Answer from the drawing. Dimensions are ordinates in mm from the lowest x, y and z of the part. Give positions to 0.01 mm unless a question says otherwise; leave off trailing zeros. Write each loop counter-clockwise with the first axis right and the second up, starting at its lowest first coordinate (ties: lowest second). Pieces come first, ordered by that corner, then holes. Notation, with made-up numbers: (-14, -8) -> (42, -8) arc R23 ccw to (42, 14) -> close; hole circle Ø3 at (-38.5, 51.5). An arc over 180 degrees is marked (long way). Write item = value, one per line.
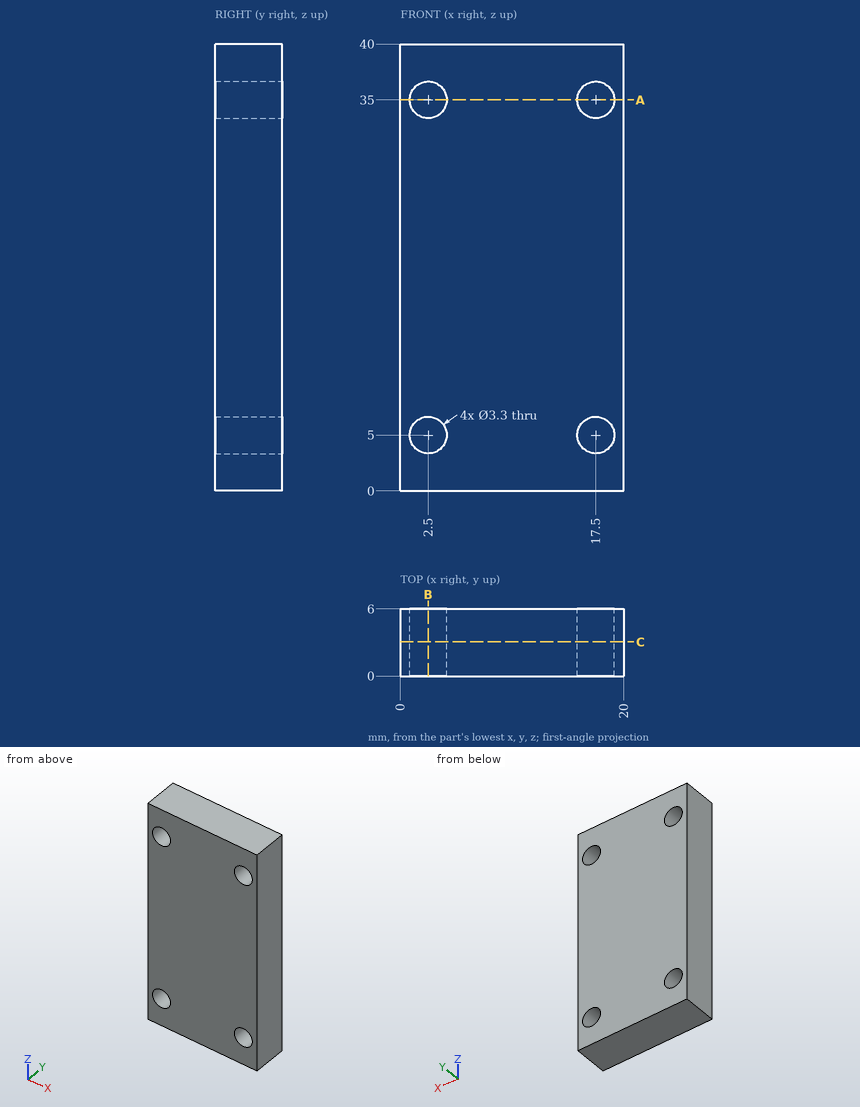
(1) Given P1, Ø8, axis at x = 4, z = 33, coming from the -Y side, flat-ended and moving along its own axis, determine where the tip first touches the part or whether it passes through.
Checks:
P1 = 0
(2) Consider L1, parallel to Z at x = 2.5, y = 3.3; L2, parallel to Z at x = 3.75, y = 4.45; L3, parallel to X at y = 3.95, z = 5.5. Determine where each line is inside the solid, lowest interval first.
Checks:
L1 = 0 to 3.35, 6.65 to 33.35, 36.65 to 40
L2 = 0 to 3.92, 6.08 to 33.92, 36.08 to 40
L3 = 0 to 0.93, 4.07 to 15.93, 19.07 to 20
(3) The part is cut by section A-A on z = 35. Determine the outline of the cut face in (x, y), plus the area to 3 significant figures.
Checks:
outline = (0, 0) -> (0.85, 0) -> (0.85, 6) -> (0, 6) -> close; (4.15, 0) -> (15.85, 0) -> (15.85, 6) -> (4.15, 6) -> close; (19.15, 0) -> (20, 0) -> (20, 6) -> (19.15, 6) -> close
area = 80.4 mm²
(4) The part is cut by section B-B on x = 2.5. Determine the outline of the cut face in (y, z).
Checks:
outline = (0, 0) -> (6, 0) -> (6, 3.35) -> (0, 3.35) -> close; (0, 6.65) -> (6, 6.65) -> (6, 33.35) -> (0, 33.35) -> close; (0, 36.65) -> (6, 36.65) -> (6, 40) -> (0, 40) -> close
(5) The part is cut by section C-C on y = 3.05. Determine the outline of the cut face in (x, z), plus the area to 3 significant figures.
Checks:
outline = (0, 0) -> (20, 0) -> (20, 40) -> (0, 40) -> close; hole circle Ø3.3 at (2.5, 5); hole circle Ø3.3 at (2.5, 35); hole circle Ø3.3 at (17.5, 5); hole circle Ø3.3 at (17.5, 35)
area = 766 mm²
